```python
from build123d import *

# Parameters (mm, degrees)
SKETCH1_W                                            = 132
SKETCH1_H                                            = 50
BOSS_EXTRUDE1_DEPTH                                  = 9
M4_TAPPED_HOLE1_D                                    = 3.3
M4_TAPPED_HOLE1_DEPTH                                = 14.008579979
M4_TAPPED_HOLE1_TIP                                  = 0.991420021
FILLET1_R                                            = 0.5
SKETCH5_R                                            = 11.1
CUT_EXTRUDE1_DEPTH                                   = 72.147733625
M5_TAPPED_HOLE1_D                                    = 4.2
CSK_FOR_M4_HEX_SOCKET_COUNTERSUNK_CAP_SC_D           = 4.5
CSK_FOR_M4_HEX_SOCKET_COUNTERSUNK_CAP_SC_CSINK_D     = 8.96
CSK_FOR_M4_HEX_SOCKET_COUNTERSUNK_CAP_SC_CSINK_ANGLE = 90
M4_TAPPED_HOLE2_D                                    = 3.3
CIRPATTERN1_COUNT                                    = 8
CUT_EXTRUDE2_DEPTH                                   = 10
CHAMFER1_SIZE                                        = 0.5
FILLET2_R                                            = 2


with BuildPart() as part:
    # Sketch1 → Boss-Extrude1 (new body)
    with BuildSketch(Plane(origin=(0, 0, 0), x_dir=(1, 0, 0), z_dir=(0, 1, 0))):
        Rectangle(SKETCH1_W, SKETCH1_H)
    extrude(amount=BOSS_EXTRUDE1_DEPTH)

    # M4 Tapped Hole1
    with Locations(Plane.ZY.offset(66)):
        with Locations((-20, 4.5), (20, 4.5)):
            Hole(M4_TAPPED_HOLE1_D / 2, depth=M4_TAPPED_HOLE1_DEPTH)
            with Locations((0, 0, -(M4_TAPPED_HOLE1_DEPTH + M4_TAPPED_HOLE1_TIP / 2))):  # 118° drill point
                Cone(0, M4_TAPPED_HOLE1_D / 2, M4_TAPPED_HOLE1_TIP, mode=Mode.SUBTRACT)

    # Fillet1
    fillet1_edges = [part.edges().sort_by_distance(p)[0] for p in [
        (-66, 4.5, 25),
        (-66, 4.5, -25),
    ]]
    fillet(fillet1_edges, radius=FILLET1_R)

    # Sketch5 → Cut-Extrude1 (cut, through all)
    with BuildSketch(Plane(origin=(0, 9, 0), x_dir=(1, 0, 0), z_dir=(0, 1, 0))):
        with Locations(Location((-41.5, 0, 0), (0, 0, 270))):
            Circle(SKETCH5_R)
    extrude(amount=-CUT_EXTRUDE1_DEPTH, mode=Mode.SUBTRACT)

    # M5 Tapped Hole1 (through all)
    with Locations(Plane(origin=(0, 9, 0), x_dir=(1, 0, 0), z_dir=(0, 1, 0))):
        with Locations((33.5, 15), (33.5, -15), (58.5, -15), (58.5, 15)):
            Hole(M5_TAPPED_HOLE1_D / 2)

    # CSK for M4 Hex Socket Countersunk Cap Screw1 (through all)
    with Locations(Plane(origin=(0, 0, 0), x_dir=(-1, 0, 0), z_dir=(0, -1, 0))):
        with Locations((1, -20), (46, -20), (46, 20), (1, 20)):
            CounterSinkHole(CSK_FOR_M4_HEX_SOCKET_COUNTERSUNK_CAP_SC_D / 2, CSK_FOR_M4_HEX_SOCKET_COUNTERSUNK_CAP_SC_CSINK_D / 2, counter_sink_angle=CSK_FOR_M4_HEX_SOCKET_COUNTERSUNK_CAP_SC_CSINK_ANGLE)

    # M4 Tapped Hole2 (through all)
    with Locations(Plane(origin=(0, 9, 0), x_dir=(1, 0, 0), z_dir=(0, 1, 0))):
        with Locations((-57.5, 0)):
            m4_tapped_hole2 = Hole(M4_TAPPED_HOLE2_D / 2)

    # CirPattern1: M4 Tapped Hole2 ×8 about axis, 2 skipped
    cirpattern1_axis = Axis((-41.5, 0, 0), (0, -1, 0))
    add([m4_tapped_hole2.rotate(cirpattern1_axis, i * 360 / CIRPATTERN1_COUNT) for i in range(1, CIRPATTERN1_COUNT) if i not in (2, 6)], mode=Mode.SUBTRACT)

    # Sketch17 → Cut-Extrude2 (cut)
    with BuildSketch(Plane(origin=(0, 9, 0), x_dir=(1, 0, 0), z_dir=(0, 1, 0))):
        with BuildLine():
            Line((66, -4.5), (66, 4.5))
            Line((66, 4.5), (48.179449472, 4.5))
            ThreePointArc((48.179449472, 4.5), (41, 0), (48.179449472, -4.5))
            Line((48.179449472, -4.5), (66, -4.5))
        make_face()
    extrude(amount=-CUT_EXTRUDE2_DEPTH, mode=Mode.SUBTRACT)

    # Sketch18 → Cut-Revolve1 (revolve, cut)
    with BuildSketch(Plane.XY):
        with BuildLine():
            Line((46, 9), (46, 1.00225345))
            ThreePointArc((46, 1.00225345), (51.841595957, 3.843776079), (55.792779203, 9))
            Line((55.792779203, 9), (46, 9))
        make_face()
    revolve(axis=Axis((46, 9, 0), (0, -1, 0)), mode=Mode.SUBTRACT)

    # Chamfer1
    # the kernel refuses this chamfer: 1.5, 0.5 mm, written as the material it takes off along each edge
    with BuildSketch(Plane(origin=(46, 9, 0), x_dir=(0.9999950652018582, 0, 0.003141587485879922), z_dir=(0.003141587485879922, 0, -0.9999950652018582))) as chamfer1_piece_1:
        with BuildLine():
            Line((9.792779203 + CHAMFER1_SIZE, 0), (8.806159122, 1.826299898))
            ThreePointArc((8.806159122, 1.826299898), (9.31899594, 0.957300628), (9.792779203, 0))
            Line((9.792779203, 0), (9.792779203 + CHAMFER1_SIZE, 0))
        make_face()
    revolve(axis=Axis((46, 9, 0), (0, -1, 0)), revolution_arc=359.64, mode=Mode.SUBTRACT)

    # Fillet2
    fillet2_edges = [part.edges().sort_by_distance(p)[0] for p in [
        (66, 4.5, 25),
        (66, 4.5, -25),
    ]]
    fillet(fillet2_edges, radius=FILLET2_R)


solid = part.part
```
The model under review builds one solid part; all positions refer to its coordinate system, in mm. A direction names the side the tool comes from. Round coordinates to 2 decimals unless told otherwise and drop trailing zeros. Loops run counter-clockwise (first coordinate to the right, second up) from the corner with the lowest first, then second, coordinate; pieces in that order, holes last. Notation, with made-up numbers: M 12,15.5 L 58,15.5 A24 cw 58,36.5 Z; hole C 84,61.25 d4. An arc over 180 degrees is marked long. Answer as a JSON object with one key per item and string values.
(1) Take a section at D-D on x = -46. Give the boundary of the cut face in (y, z), and give its area (3 significant figures).
Resolved:
{"outline": "M 0,-25 L 9,-25 L 9,-22.25 L 2.23,-22.25 L 0,-24.48 Z; M 0,-15.52 L 2.23,-17.75 L 9,-17.75 L 9,-10.15 L 0,-10.15 Z; M 0,10.15 L 9,10.15 L 9,17.75 L 2.23,17.75 L 0,15.52 Z; M 0,24.48 L 2.23,22.25 L 9,22.25 L 9,25 L 0,25 Z", "area": "176 mm²"}
(2) Draft analysis for pull direction Z (two halves, no side actions). For faces 4 (the flat face through (66, 4, -14)), 5 (the cylindrical face through (-55.85, 4.44, -0.07)), 6 (the flat face through (-2, 4, -25)), state which applies: released by +Z, released by -Z, zero draft, split by the parting line, or undercut.
Resolved:
{"face 4": "zero draft", "face 5": "undercut", "face 6": "released by -Z"}
(3) Clearance check with flat-ended pins moving along their axes: P1, Ø3, axis at y = 4.5, z = 20, coming from the -X side; P2, Ø2.5, axis at y = 4.5, z = -20, coming from the -X side; P3, Ø6, axis at x = 45.5, z = 6, coming from the +Y side. State where each tip first meets the part, or that it passes through.
Resolved:
{"P1": "x = -51.9", "P2": "x = -51.75", "P3": "y = 7.44"}
(4) Take a section at B-B on x = -25.5. Give the boundary of the cut face in (y, z).
Resolved:
{"outline": "M 0,-25 L 9,-25 L 9,-1.65 L 0,-1.65 Z; M 0,1.65 L 9,1.65 L 9,25 L 0,25 Z"}
(5) To check wall thickness, follow line 1 along X through (y, z) = (3.75, 11.5); line 2 along Z through (x, y) = (58.5, 5); line 3 along Z through (x, y) = (-2.5, 2.25). State the ranges of each line that lie inside material, in increasing order.
Resolved:
{"line 1": "-66 to -54.45, -51.17 to -31.83, -28.55 to 66", "line 2": "-25 to -17.1, -12.9 to -4.5, 4.5 to 12.9, 17.1 to 25", "line 3": "-25 to -21.68, -18.32 to 18.32, 21.68 to 25"}
(6) Take a section at C-C on z = 0. Count the separate pieces of the cut face and the enclosed holes in it, and give its area (3 significant figures).
Resolved:
{"separate pieces": "4", "enclosed holes": "0", "area": "687 mm²"}
(7) Tool access review of faces 1 (the cylindrical face through (-58.9, 3.5, -18.69)), 2 (the cylindrical face through (-47.786, 5.662, -18.631)), 3 (the flat face through (59, 5, -4.5)): name each direction out of +Z, -Z, +X, -X, +Y, -Y from which nothing blocks a thin tool from reaching the whole face with its end or side.
Resolved:
{"face 1": "-X", "face 2": "+Y, -Y", "face 3": "+X, +Y, -Y"}
(8) Take a section at A-A on x = 58.5. Give the boundary of the cut face in (y, z).
Resolved:
{"outline": "M 0,-25 L 9,-25 L 9,-17.1 L 0,-17.1 Z; M 0,-12.9 L 9,-12.9 L 9,-4.5 L 0,-4.5 Z; M 0,4.5 L 9,4.5 L 9,12.9 L 0,12.9 Z; M 0,17.1 L 9,17.1 L 9,25 L 0,25 Z"}
